Part print with two shaded views. Sizes in mm from the minimum x, y, z corner. A direction names the side the tool comes from. Round coordinates to 2 decimals unless told otherwise and drop trailing zeros. Loops run counter-clockwise (first coordinate to the right, second up) from the corner with the lowest first, then second, coordinate; pieces in that order, holes last. Notation, with made-up numbers: (-3, 50) -> (22, 50) arc R31 cw to (22, 88) -> close; hole circle Ø7 at (-12, -40). An arc over 180 degrees is marked (long way). Use a Markdown table: item, result. Add a question column.
Item 1: Cut at D-D, the plane y = 7. List the corners of the cut face in (x, z).
Item 2: Cut at B-B, the plane z = 13. List the corners of the cut face in (x, y).
Item 3: Which spindle directions (+Z, -Z, +X, -X, +Y, -Y) get a long thin tool onto all of the face, cutting with end or side? Do the marked faces 1 and 2. Say none if no direction does.
Item 4: Two-plate mould, pull along Y, no slides. Class the marked faces 3, 4 and 5: pulls with the +Y half, pulls with the -Y half, needs draft (parallel to the pull), parting line crosses it, or undercut.
Item 5: Cut at C-C, the plane x = 15. List the corners of the cut face in (y, z), plus the area to 3 significant figures.
Item 6: Cut at A-A, the plane y = 17. List the corners of the cut face in (x, z).
Item 7: Probe line 1 (Z direction, x = 3.5, y = 29); line 2 (Y direction, x = 1, z = 16); line 3 (Y direction, x = 4, z = 31.5). List the from-to ranges inside material, lowest first. Write a range as [from, to].
Item 8: Flat gauge pins, fed straight in: pin 1 (7 mm diameter, centred on y = 15, z = 19.5, fed in from -X); pin 2 (3 mm diameter, centred on x = 8.5, y = 5.5, fed in from +Z); pin 3 (0.9 mm diameter, centred on y = 36, z = 19, fed in from +X). Where does each tip first touch, or does it go through?
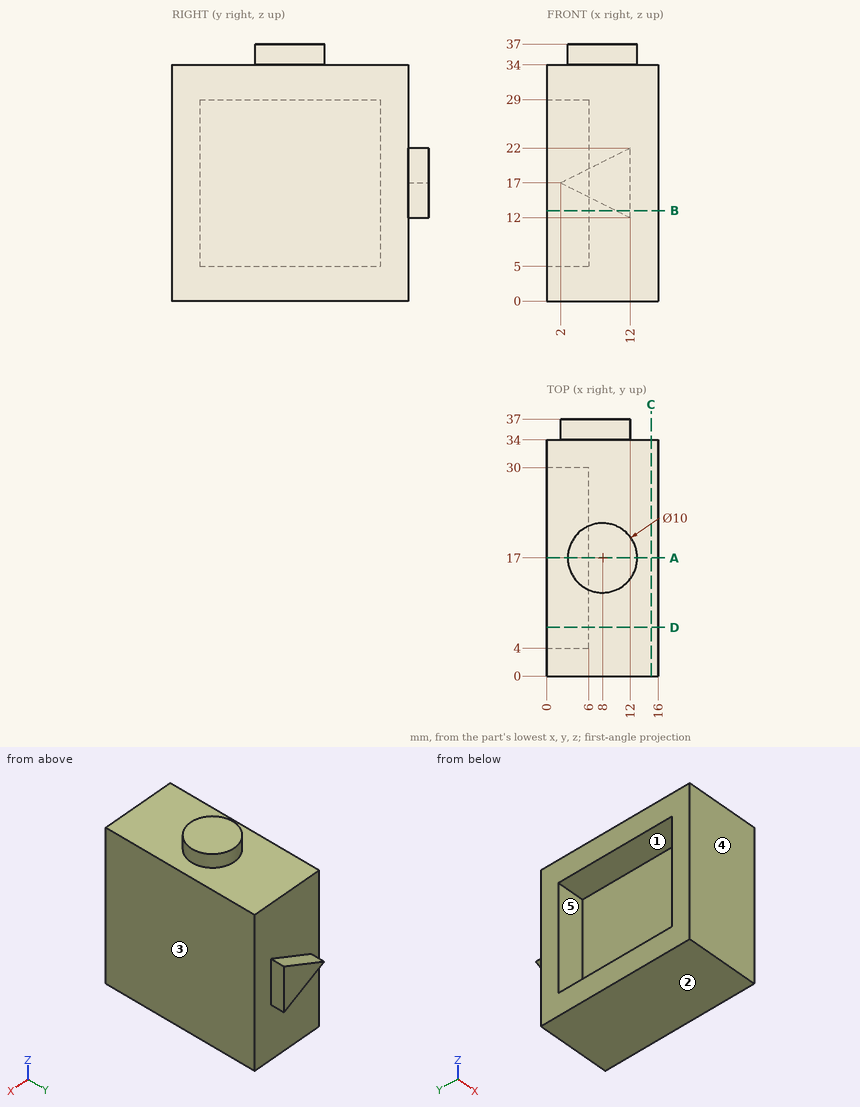
A:
| question | item | result |
|---|---|---|
| 1 | outline | (0, 0) -> (16, 0) -> (16, 34) -> (0, 34) -> (0, 29) -> (6, 29) -> (6, 5) -> (0, 5) -> close |
| 2 | outline | (0, 0) -> (16, 0) -> (16, 34) -> (12, 34) -> (12, 37) -> (10, 37) -> (10, 34) -> (0, 34) -> (0, 30) -> (6, 30) -> (6, 4) -> (0, 4) -> close |
| 3 | face 1 | -X |
| 3 | face 2 | -Z, +X, -X, +Y, -Y |
| 4 | face 3 | needs draft |
| 4 | face 4 | pulls with the -Y half |
| 4 | face 5 | undercut |
| 5 | outline | (0, 0) -> (34, 0) -> (34, 34) -> (0, 34) -> close |
| 5 | area | 1,160 mm^2 |
| 6 | outline | (0, 0) -> (16, 0) -> (16, 34) -> (13, 34) -> (13, 37) -> (3, 37) -> (3, 34) -> (0, 34) -> (0, 29) -> (6, 29) -> (6, 5) -> (0, 5) -> close |
| 7 | line 1 | z = [0, 5], [29, 34] |
| 7 | line 2 | y = [0, 4], [30, 34] |
| 7 | line 3 | y = [0, 34] |
| 8 | pin 1 | stops at x = 6 |
| 8 | pin 2 | stops at z = 34 |
| 8 | pin 3 | stops at x = 12 |
